```python
from build123d import *

# Parameters (mm, degrees)
BOSS_EXTRUDE1_DEPTH = 30
FILLET1_R           = 0.8
SKETCH3_R           = 3
CUT_EXTRUDE1_DEPTH  = 9
SKETCH4_R           = 1.55
CUT_EXTRUDE2_DEPTH  = 37.426390381
FILLET2_R           = 5


with BuildPart() as part:
    # Sketch1 → Boss-Extrude1 (new body)
    with BuildSketch(Plane.XY):
        with BuildLine():
            Line((0, 0), (17.5, 0))
            Line((17.5, 0), (17.5, 9.44))
            Line((17.5, 9.44), (15.025126266, 11.914873734))
            ThreePointArc((15.025126266, 11.914873734), (4.907782078, 9.219443047), (7.603212766, 19.336787234))
            Line((7.603212766, 19.336787234), (5.128339032, 21.811660968))
            Line((5.128339032, 21.811660968), (0, 16.683321936))
            Line((0, 16.683321936), (0, 0))
        make_face()
    extrude(amount=BOSS_EXTRUDE1_DEPTH)

    # Fillet1
    fillet1_edges = [part.edges().sort_by_distance(p)[0] for p in [
        (7.603212766, 19.336787234, 15),
        (15.025126266, 11.914873734, 15),
    ]]
    fillet(fillet1_edges, radius=FILLET1_R)

    # Sketch3 → Cut-Extrude1 (cut)
    with BuildSketch(Plane(origin=(0, 10.828405067, 0), x_dir=(-1, 0, 0), z_dir=(0, -1, 0))):
        with Locations(Location((-8.875495285, -5, 0), (0, 0, 270))):
            Circle(SKETCH3_R)
        with Locations(Location((-8.875495285, -25, 0), (0, 0, 270))):
            Circle(SKETCH3_R)
    extrude(amount=CUT_EXTRUDE1_DEPTH, mode=Mode.SUBTRACT)

    # Sketch4 → Cut-Extrude2 (cut, through all)
    with BuildSketch(Plane(origin=(0, 10.828405067, 0), x_dir=(-1, 0, 0), z_dir=(0, -1, 0))):
        with Locations(Location((-8.875495285, -5, 0), (0, 0, 90))):
            Circle(SKETCH4_R)
        with Locations(Location((-8.875495285, -25, 0), (0, 0, 90))):
            Circle(SKETCH4_R)
    extrude(amount=CUT_EXTRUDE2_DEPTH, mode=Mode.SUBTRACT)

    # Fillet2
    fillet2_edges = [part.edges().sort_by_distance(p)[0] for p in [
        (0, 16.683321936, 15),
    ]]
    fillet(fillet2_edges, radius=FILLET2_R)


solid = part.part
```
For this review, take the finished solid that the model builds, in its own axes (mm). A direction names the side the tool comes from. Round coordinates to 2 decimals unless told otherwise and drop trailing zeros. Write each loop counter-clockwise with the first axis right and the second up, starting at its lowest first coordinate (ties: lowest second). Pieces come first, ordered by that corner, then holes. Notation, with made-up numbers: (88.5, 83) - (122.5, 83) arc R11 cw to (122.5, 93) - close; hole circle Ø5 at (72, 58.25). An arc over 180 degrees is marked (long way). Use CSV: the item, a comma, the result in double quotes.
1) Add section B-B on z = 5. Write out the cut boundary in (x, y).
Conclusion:
outline,"(0, 0) - (7.33, 0) - (7.33, 1.83) - (5.88, 1.83) - (5.88, 8.43) arc R6.05 cw to (6.52, 18.93) arc R0.8 ccw to (6.73, 20.21) - (5.13, 21.81) - (1.46, 18.15) arc R5 ccw to (0, 14.61) - close; (10.43, 0) - (17.5, 0) - (17.5, 9.44) - (15.9, 11.04) arc R0.8 ccw to (14.62, 10.83) arc R6.05 cw to (11.88, 8.08) - (11.88, 1.83) - (10.43, 1.83) - close"
2) Add section D-D on x = 15.5. Write out the cut boundary in (y, z), and give its area (3 significant figures).
Conclusion:
outline,"(0, 0) - (11.26, 0) - (11.26, 30) - (0, 30) - close"
area,"338 mm^2"
3) The part is to be moulded in two halves that separate along Z. For faces 1 (the cylindrical face through (15.213, 11.266, 15.21)), 2 (the cylindrical face through (5.9, 5.18, 24.61)), 3 (the flat face through (7, 6, 0)), 4 (the flat face through (7, 6, 30)), say which applies: pulls with the +Z half, pulls with the -Z half, needs draft (parallel to the pull), parting line crosses it, or undercut.
Conclusion:
face 1,"needs draft"
face 2,"undercut"
face 3,"pulls with the -Z half"
face 4,"pulls with the +Z half"
4) Clearance check with flat-ended pins moving along their axes: pin 1 Ø6 at (y, z) = (14.5, 25) entering from +X; pin 2 Ø3 at (y, z) = (19.5, 24.5) entering from -X; pin 3 Ø2 at (x, z) = (11, 27) entering from +Y; pin 4 Ø2.5 at (x, z) = (8.88, 25) entering from +Y. State where each tip first meets the part, or that it passes through.
Conclusion:
pin 1,"stops at x = 4.65"
pin 2,"stops at x = 1.32"
pin 3,"stops at y = 8.14"
pin 4,"passes through"
5) For faces 5 (the cylindrical face through (9.923, 0.927, 6.142)), 6 (the flat face through (10.2, 1.828, 6.3)), list the 3-axis set-ups (+Z, -Z, +X, -X, +Y, -Y) from which the entire face can be reached by the end or side of a thin tool; tool diameter is ignored.
Conclusion:
face 5,"+Y, -Y"
face 6,"none"
6) Wall thickness on line 1 along X through (y, z) = (5.5, 5); line 2 along Z through (x, y) = (9.5, 6.5); line 3 along X through (y, z) = (1.25, 5): over which ranges is each line inside the solid? List them lowest first. Write a range as from..to.
Conclusion:
line 1,"x = 0..5.88, 11.88..17.5"
line 2,"z = 0..2.07, 7.93..22.07, 27.93..30"
line 3,"x = 0..7.33, 10.43..17.5"
7) Add section A-A on z = 11. Write out the cut boundary in (x, y).
Conclusion:
outline,"(0, 0) - (17.5, 0) - (17.5, 9.44) - (15.9, 11.04) arc R0.8 ccw to (14.62, 10.83) arc R6.05 cw (long way) to (6.52, 18.93) arc R0.8 ccw to (6.73, 20.21) - (5.13, 21.81) - (1.46, 18.15) arc R5 ccw to (0, 14.61) - close"
8) Add section C-C on y = 4. Write out the cut boundary in (x, z).
Conclusion:
outline,"(0, 0) - (17.5, 0) - (17.5, 30) - (0, 30) - close; hole circle Ø6 at (8.88, 5); hole circle Ø6 at (8.88, 25)"
